Design review of the part built by this model. Coordinates are the model's own, in mm. Round coordinates to 2 decimals unless told otherwise and drop trailing zeros. Order: outer loops, then holes, each group sorted by start corner. A loop starts at its lowest first (then second) coordinate and runs counter-clockwise, first axis right, second up. Notation, with made-up numbers: (52, -19) - (96, -19) arc R12 cw to (96, -7) - close; hole circle Ø3 at (-8, 55.25). An arc over 180 degrees is marked (long way). Write item = value, one per line.
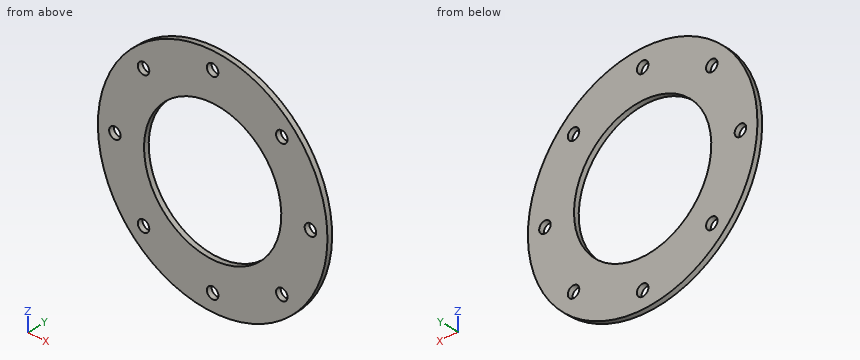
from build123d import *

# Parameters (mm, degrees)
SKETCH1_R             = 135
SKETCH1_R_2           = 80.75
BOSS_EXTRUDE1_DEPTH   = 6
M12_CLEARANCE_HOLE1_D = 13.5


with BuildPart() as part:
    # Sketch1 → Boss-Extrude1 (new body)
    with BuildSketch(Plane(origin=(0, 0, 0), x_dir=(1, 0, 0), z_dir=(0, 1, 0))):
        with Locations(Location((0, 0, 0), (0, 0, 270))):
            Circle(SKETCH1_R)
        with Locations(Location((0, 0, 0), (0, 0, 270))):
            Circle(SKETCH1_R_2, mode=Mode.SUBTRACT)
    extrude(amount=BOSS_EXTRUDE1_DEPTH)

    # M12 Clearance Hole1 (through all)
    with Locations(Plane(origin=(0, 6, 0), x_dir=(1, 0, 0), z_dir=(0, 1, 0))):
        with Locations((0, 115), (81.317279836, 81.317279836), (115, 0), (81.317279836, -81.317279836), (0, -115), (-81.317279836, -81.317279836), (-115, 0), (-81.317279836, 81.317279836), (0, 0)):
            Hole(M12_CLEARANCE_HOLE1_D / 2)


solid = part.part
1) Clearance check with flat-ended pins moving along their axes: pin 1 Ø2 at (y, z) = (1.5, 48) entering from -X; pin 2 Ø4 at (x, z) = (60, -48) entering from +Y. State where each tip first meets the part, or that it passes through.
Findings:
pin_1 = -126.55
pin_2 = through
2) We need section D-D on z = 67. Write out the cut boundary in (x, y), and give its area (3 significant figures).
Findings:
outline = (-117.2, 0) - (-45.07, 0) - (-45.07, 6) - (-117.2, 6) - close; (45.07, 0) - (117.2, 0) - (117.2, 6) - (45.07, 6) - close
area = 866 mm^2
3) We need section C-C on x = -115. Write out the cut boundary in (y, z).
Findings:
outline = (0, -70.71) - (6, -70.71) - (6, -6.75) - (0, -6.75) - close; (0, 6.75) - (6, 6.75) - (6, 70.71) - (0, 70.71) - close
4) We need section B-B on x = 0. Write out the cut boundary in (y, z).
Findings:
outline = (0, -135) - (6, -135) - (6, -121.75) - (0, -121.75) - close; (0, -108.25) - (6, -108.25) - (6, -80.75) - (0, -80.75) - close; (0, 80.75) - (6, 80.75) - (6, 108.25) - (0, 108.25) - close; (0, 121.75) - (6, 121.75) - (6, 135) - (0, 135) - close
5) To check wall thickness, follow L1, parallel to X at y = 1.8, z = 113; L2, parallel to Z at x = -110.5, y = 4.8; L3, parallel to Z at x = 44.5, y = 1. State the ranges of each line that lie inside material, in increasing order. Write a range as from..to.
Findings:
L1 = -73.86..-6.45, 6.45..73.86
L2 = -77.55..-5.03, 5.03..77.55
L3 = -127.45..-67.38, 67.38..127.45
6) We need section A-A on z = 0. Write out the cut boundary in (x, y).
Findings:
outline = (-135, 0) - (-121.75, 0) - (-121.75, 6) - (-135, 6) - close; (-108.25, 0) - (-80.75, 0) - (-80.75, 6) - (-108.25, 6) - close; (80.75, 0) - (108.25, 0) - (108.25, 6) - (80.75, 6) - close; (121.75, 0) - (135, 0) - (135, 6) - (121.75, 6) - close
